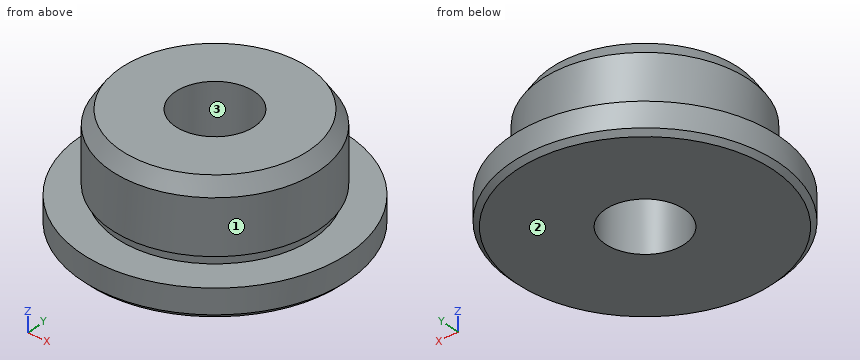
```python
from build123d import *

# Parameters (mm, degrees)
F2_SIZE2 = 1
F2_SIZE  = 1.5
F3_SIZE  = 0.5
F4_W     = 0.5
F4_H     = 1


with BuildPart() as f1:
    # F0 (on Front) → F1 (revolve)
    with BuildSketch(Plane.XZ):
        Polygon((10.5, 11), (4, 11), (4, 0), (13.5, 0), (13.5, 3), (10.5, 3), align=None)
    revolve(axis=Axis((0, 0, 2.786824197), (0, 0, 1)))

    # F2
    f2_edges = [f1.edges().sort_by_distance(p)[0] for p in [
        (-10.5, 0, 11),
    ]]
    f2_side = f1.faces().sort_by_distance((-10.5, 0, 7))[0]
    chamfer(f2_edges, length=F2_SIZE, length2=F2_SIZE2, reference=f2_side)

    # F3
    f3_edges = [f1.edges().sort_by_distance(p)[0] for p in [
        (-13.5, 0, 0),
    ]]
    chamfer(f3_edges, length=F3_SIZE)

    # F4 (on Front) → F5 (revolve, cut)
    with BuildSketch(Plane.XZ):
        with Locations((10.25, 3.5)):
            Rectangle(F4_W, F4_H)
    revolve(axis=Axis((0, 0, 2.786824197), (0, 0, 1)), mode=Mode.SUBTRACT)


solid = f1.part
```
Work out the finished part from the listing and answer in its coordinate system (mm). Face numbers are marked on the shaded views. Coordinates: 2 decimals unless noted, no trailing zeros. Loops run counter-clockwise (first coordinate to the right, second up) from the corner with the lowest first, then second, coordinate; pieces in that order, holes last. Notation, with made-up numbers: M 12,42 L 41,42 A6 ccw 41,50 Z; hole C 8.25,14 d8. An arc over 180 degrees is marked long. Use CSV: the item, a comma, the result in double quotes. Start each with the question number.
(1) Find section A-A, the plane x = 0. Give the vertices of the cut face in (y, z), then the cut area to 3 significant figures.
(2) Consider line 1 (Y direction, x = 0, z = 6.75); line 2 (Y direction, x = -0.25, z = 0.5); line 3 (Z direction, x = 10, y = -4.25). Determine where each line is inside the solid, lowest interval first.
(3) For a pull along Y with two mould halves and no side action, classify the marked faces 1, 2 and 3 as +Y half, -Y half, draft (parallel to the pull), parting line (faces both ways), or undercut.
(4) Find section C-C, the plane z = 7.5. Give the vertices of the cut face in (x, y).
(5) Given pin 1 Ø2 at (y, z) = (-7, 7) entering from -X; pin 2 Ø5 at (y, z) = (5.5, 7.5) entering from -X; pin 3 Ø5 at (y, z) = (-8, 7) entering from -X, each flat-ended and moving along its own axis, determine where each tip first touches the part or whether it passes through.
(6) Find section D-D, the plane z = 10. Give the vertices of the cut face in (x, y), then the cut area to 3 significant figures.
Recorded:
1,outline,"M -13.5,0.5 L -13,0 L -4,0 L -4,11 L -9.5,11 L -10.5,9.5 L -10.5,4 L -10,4 L -10,3 L -13.5,3 Z; M 4,0 L 13,0 L 13.5,0.5 L 13.5,3 L 10,3 L 10,4 L 10.5,4 L 10.5,9.5 L 9.5,11 L 4,11 Z"
1,area,"158 mm^2"
2,line 1,"y = -10.5 to -4, 4 to 10.5"
2,line 2,"y = -13.5 to -3.99, 3.99 to 13.5"
2,line 3,"z = 0 to 3"
3,face 1,"parting line"
3,face 2,"draft"
3,face 3,"undercut"
4,outline,"C 0,0 d21; hole C 0,0 d8"
5,pin 1,"stops at x = -8.62"
5,pin 2,"stops at x = -10.06"
5,pin 3,"stops at x = -8.94"
6,outline,"C 0,0 d20.33; hole C 0,0 d8"
6,area,"274 mm^2"
